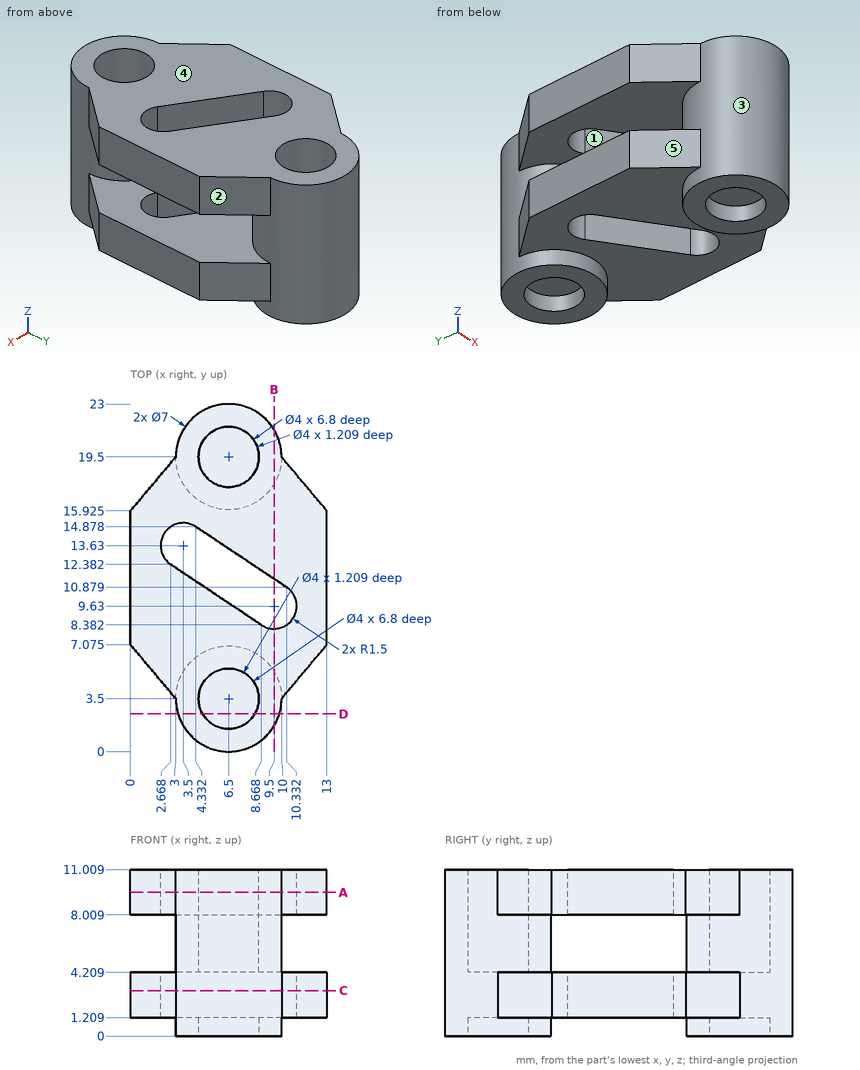
For this review, use the dimensioned drawing (mm, ordinates from the lowest corner) and the shaded views. A direction names the side the tool comes from. Coordinates: 2 decimals unless noted, no trailing zeros. Order: outer loops, then holes, each group sorted by start corner. A loop starts at its lowest first (then second) coordinate and runs counter-clockwise, first axis right, second up. Notation, with made-up numbers: M 9,45 L 61,45 A20 ccw 61,71 Z; hole C 23.5,64.5 d8. An arc over 180 degrees is marked long. Answer as a JSON object with one key per item and string values. Group by question number.
1) Mouldability with a two-part tool opening along Y and no side actions: class the marked faces 3, 4 and 5 as pulls with the +Y half, pulls with the -Y half, needs draft (parallel to the pull), parting line crosses it, or undercut.
2) Add section D-D, the plane y = 2.5. Write out the cut boundary in (x, z) (1 decimal).
3) For pin 1 (2.5 mm diameter, centred on x = 6.5, y = 19.5, fed in from +Z); pin 2 (1.5 mm diameter, centred on x = 11.5, y = 16.5, fed in from -Z); pin 3 (5 mm diameter, centred on x = 10, z = 6, fed in from +Y) (1 decimal), all flat-tipped, find the tip position at first contact; note any pin that passes through.
4) Add section B-B, the plane x = 9.5. Write out the cut boundary in (y, z), then the cut area to 3 significant figures.
5) Add section A-A, the plane z = 9.5. Write out the cut boundary in (x, y) (1 decimal).
6) Tool access review of the marked faces 1 and 2: name each direction out of +Z, -Z, +X, -X, +Y, -Y from which nothing blocks a thin tool from reaching the whole face with its end or side.
7) Wall thickness on L1, parallel to Y at x = 6.5, z = 0.3; L2, parallel to Z at x = 2, y = 15.75; L3, parallel to X at y = 3.5, z = 0.85: over which ranges is each line inside the solid? List them lowest first.
8) Add section C-C, the plane z = 3. Write out the cut boundary in (x, y) (1 decimal).
Computed values:
{
 "1": {"face 3": "undercut", "face 4": "needs draft", "face 5": "pulls with the -Y half"},
 "2": {"outline": "M 3.1,0 L 4.8,0 L 4.8,1.2 L 8.2,1.2 L 8.2,0 L 9.9,0 L 9.9,11 L 8.2,11 L 8.2,4.2 L 4.8,4.2 L 4.8,11 L 3.1,11 Z"},
 "3": {"pin 1": "stops at z = 4.21", "pin 2": "stops at z = 1.21", "pin 3": "stops at y = 22.9"},
 "4": {"outline": "M 1.7,0 L 5.3,0 L 5.3,1.21 L 8.13,1.21 L 8.13,4.21 L 5.3,4.21 L 5.3,8.01 L 8.13,8.01 L 8.13,11.01 L 1.7,11.01 Z; M 11.43,1.21 L 17.7,1.21 L 17.7,0 L 21.3,0 L 21.3,11.01 L 11.43,11.01 L 11.43,8.01 L 17.7,8.01 L 17.7,4.21 L 11.43,4.21 Z", "area": "134 mm^2"},
 "5": {"outline": "M 0,7.1 L 3,3.5 A3.5 ccw 10,3.5 L 13,7.1 L 13,15.9 L 10,19.5 A3.5 ccw 3,19.5 L 0,15.9 Z; hole M 2.7,12.4 L 8.7,8.4 A1.5 ccw 10.3,10.9 L 4.3,14.9 A1.5 ccw Z; hole C 6.5,3.5 d4; hole C 6.5,19.5 d4"},
 "6": {"face 1": "+Z, -Z", "face 2": "+Z, -Z, +X, +Y"},
 "7": {"L1": "y = 0 to 1.5, 5.5 to 7, 16 to 17.5, 21.5 to 23", "L2": "z = 1.21 to 4.21, 8.01 to 11.01", "L3": "x = 3 to 4.5, 8.5 to 10"},
 "8": {"outline": "M 0,7.1 L 3,3.5 A3.5 ccw 10,3.5 L 13,7.1 L 13,15.9 L 10,19.5 A3.5 ccw 3,19.5 L 0,15.9 Z; hole M 2.7,12.4 L 8.7,8.4 A1.5 ccw 10.3,10.9 L 4.3,14.9 A1.5 ccw Z"}
}
